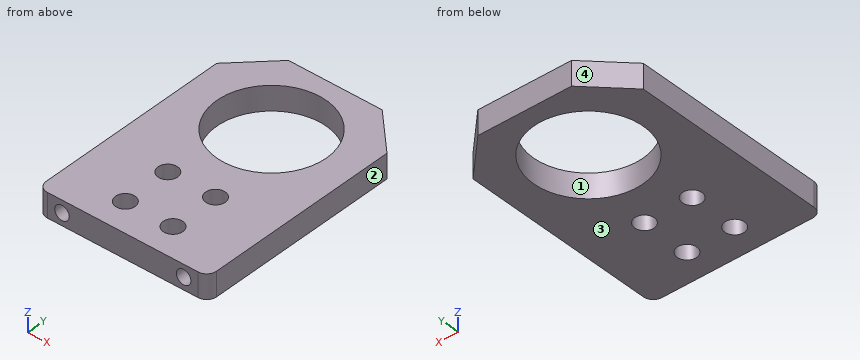
from build123d import *

# Parameters (mm, degrees)
SKETCH1_W                      = 44.45
SKETCH1_H                      = 63.5
BOSS_EXTRUDE1_DEPTH            = 3.175
CHAMFER1_SIZE                  = 10
SKETCH2_R                      = 14.2875
CUT_EXTRUDE1_DEPTH             = 40.272581084
TAP_DRILL_FOR_10_24_TAP1_D     = 3.7973
TAP_DRILL_FOR_10_24_TAP1_DEPTH = 19.05
TAP_DRILL_FOR_10_24_TAP1_TIP   = 1.140824014
F_10_CLEARANCE_HOLE1_D         = 5.1054
F_10_CLEARANCE_HOLE1_DEPTH     = 12.7
F_10_CLEARANCE_HOLE1_TIP       = 1.533816902
FILLET1_R                      = 2.54


with BuildPart() as part:
    # Sketch1 → Boss-Extrude1 (new, symmetric)
    with BuildSketch(Plane.XY):
        Rectangle(SKETCH1_W, SKETCH1_H)
    extrude(amount=BOSS_EXTRUDE1_DEPTH, both=True)

    # Chamfer1
    chamfer1_edges = [part.edges().sort_by_distance(p)[0] for p in [
        (-22.225, 31.75, 0),
        (22.225, 31.75, 0),
    ]]
    chamfer(chamfer1_edges, length=CHAMFER1_SIZE)

    # Sketch2 → Cut-Extrude1 (cut, through all)
    with BuildSketch(Plane.XY.offset(3.175)):
        with Locations((0, 12.7)):
            Circle(SKETCH2_R)
    extrude(amount=-CUT_EXTRUDE1_DEPTH, mode=Mode.SUBTRACT)

    # Tap Drill for #10-24 Tap1
    with Locations(Plane(origin=(0, -31.75, 0), x_dir=(-1, 0, 0), z_dir=(0, -1, 0))):
        with Locations((15.875, 0), (-15.875, 0)):
            Hole(TAP_DRILL_FOR_10_24_TAP1_D / 2, depth=TAP_DRILL_FOR_10_24_TAP1_DEPTH)
            with Locations((0, 0, -(TAP_DRILL_FOR_10_24_TAP1_DEPTH + TAP_DRILL_FOR_10_24_TAP1_TIP / 2))):  # 118° drill point
                Cone(0, TAP_DRILL_FOR_10_24_TAP1_D / 2, TAP_DRILL_FOR_10_24_TAP1_TIP, mode=Mode.SUBTRACT)

    # #10 Clearance Hole1
    with Locations(Plane.XY.offset(3.175)):
        with Locations((-6.223, -11.176), (6.223, -11.176), (6.223, -23.876), (-6.223, -23.876)):
            Hole(F_10_CLEARANCE_HOLE1_D / 2, depth=F_10_CLEARANCE_HOLE1_DEPTH)
            with Locations((0, 0, -(F_10_CLEARANCE_HOLE1_DEPTH + F_10_CLEARANCE_HOLE1_TIP / 2))):  # 118° drill point
                Cone(0, F_10_CLEARANCE_HOLE1_D / 2, F_10_CLEARANCE_HOLE1_TIP, mode=Mode.SUBTRACT)

    # Fillet1
    fillet1_edges = [part.edges().sort_by_distance(p)[0] for p in [
        (22.225, -31.75, 0),
        (-22.225, -31.75, 0),
    ]]
    fillet(fillet1_edges, radius=FILLET1_R)


solid = part.part
Source: CAD feature listing. Evaluate the final solid. Frame: model axes, mm. Face numbers are marked on the shaded views. Round coordinates to 2 decimals unless told otherwise and drop trailing zeros. Loops run counter-clockwise (first coordinate to the right, second up) from the corner with the lowest first, then second, coordinate; pieces in that order, holes last.
Q1. Ray query, line 1 (X direction, y = 12.5, z = -1.25) (3 decimals); line 2 (Y direction, x = 0, z = -0.5); line 3 (Y direction, x = 4, z = -2.25). Return the intervals inside material, ascending.
Q2. Section D-D, the plane x = -7.5. Return loops of the section in (y, z) (3 decimals), plus the area to 3 significant figures.
Q3. Section A-A, the plane y = -25.5. Return loops of the section in (x, z) (1 decimal).
Q4. Mould query, pull axis X, two halves, no side actions, for the marked faces 1, 2, 3 and 4. Classes: pulls with the +X half, pulls with the -X half, needs draft (parallel to the pull), parting line crosses it, or undercut.
Q5. Section C-C, the plane y = 12.7. Return loops of the section in (x, z) (1 decimal).
Q6. First-contact query: P1, Ø6, axis at x = 6.223, y = -11.176, coming from the +Z side (3 decimals). Flat tip, straight axial feed; report the tip coordinate or a pass-through.
Solutions:
1. line 1: x = -22.225 to -14.286, 14.286 to 22.225
1. line 2: y = -31.75 to -1.59, 26.99 to 31.75
1. line 3: y = -31.75 to -25.13, -22.62 to -12.43, -9.92 to -1.02, 26.42 to 31.75
2. outline: (-31.75, -3.175) - (-26.086, -3.175) - (-26.086, 3.175) - (-31.75, 3.175) - close; (-21.666, -3.175) - (-13.386, -3.175) - (-13.386, 3.175) - (-21.666, 3.175) - close; (-8.966, -3.175) - (0.539, -3.175) - (0.539, 3.175) - (-8.966, 3.175) - close; (24.861, -3.175) - (31.75, -3.175) - (31.75, 3.175) - (24.861, 3.175) - close
2. area: 193 mm2
3. outline: (-22.2, -3.2) - (-8.2, -3.2) - (-8.2, 3.2) - (-22.2, 3.2) - close; (-4.3, -3.2) - (4.3, -3.2) - (4.3, 3.2) - (-4.3, 3.2) - close; (8.2, -3.2) - (22.2, -3.2) - (22.2, 3.2) - (8.2, 3.2) - close; hole circle Ø3.8 at (-15.9, 0); hole circle Ø3.8 at (15.9, 0)
4. face 1: undercut
4. face 2: pulls with the +X half
4. face 3: needs draft
4. face 4: pulls with the -X half
5. outline: (-22.2, -3.2) - (-14.3, -3.2) - (-14.3, 3.2) - (-22.2, 3.2) - close; (14.3, -3.2) - (22.2, -3.2) - (22.2, 3.2) - (14.3, 3.2) - close
6. P1: stops at z = 3.175
